Here's how the part is built. I have some questions about the finished solid (model axes, mm). A direction names the side the tool comes from. Round coordinates to 2 decimals unless told otherwise and drop trailing zeros. Order: outer loops, then holes, each group sorted by start corner. A loop starts at its lowest first (then second) coordinate and runs counter-clockwise, first axis right, second up.
```python
from build123d import *

# Parameters (mm, degrees)
CORTAR_EXTRUIR1_REACH   = 95.608
CROQUIS2_R              = 3.5
CROQUIS3_R              = 7
CROQUIS3_R_2            = 3.5
SALIENTE_EXTRUIR1_DEPTH = 6
SALIENTE_EXTRUIR2_START = 3
CROQUIS4_R              = 60.229990605
CROQUIS4_R_2            = 3.5
SALIENTE_EXTRUIR2_DEPTH = 3
CROQUIS5_R              = 5.5
CORTAR_EXTRUIR2_DEPTH   = 6.5
CORTAR_EXTRUIR3_REACH   = 96.128
CORTAR_EXTRUIR4_DEPTH   = 3
CHAFL_N1_SIZE           = 1.5
REDONDEO1_R             = 3


with BuildPart() as part:
    # Croquis1 → Revolución1 (revolve)
    with BuildSketch(Plane.XY, mode=Mode.PRIVATE) as revoluci_n1_sk:
        Polygon((-65.360292755, 76.904610688), (-65.360292755, 76.220570402), (-63.480907514, 76.220570402), (-58.829575529, 89), (0, 89), (0, 91), (-60.229990605, 91), align=None)
    revolve(revoluci_n1_sk.sketch.rotate(Axis((0, 89, 0), (0, 1, 0)), 270), axis=Axis((0, 89, 0), (0, 1, 0)))

    # Croquis2 → Cortar-Extruir1 (cut, up to next)
    with BuildSketch(Plane(origin=(0, 91, 0), x_dir=(1, 0, 0), z_dir=(0, 1, 0)), mode=Mode.PRIVATE) as cortar_extruir1_sk1:
        with Locations(Location((32, 0, 0), (0, 0, 270))):
            Circle(CROQUIS2_R)
    cortar_extruir1_tool1 = extrude(cortar_extruir1_sk1.sketch, amount=-CORTAR_EXTRUIR1_REACH, mode=Mode.PRIVATE) & part.part
    # Croquis2 → Cortar-Extruir1 (cut, up to next)
    with BuildSketch(Plane(origin=(0, 91, 0), x_dir=(1, 0, 0), z_dir=(0, 1, 0)), mode=Mode.PRIVATE) as cortar_extruir1_sk2:
        with Locations(Location((-32, 0, 0), (0, 0, 270))):
            Circle(CROQUIS2_R)
    cortar_extruir1_tool2 = extrude(cortar_extruir1_sk2.sketch, amount=-CORTAR_EXTRUIR1_REACH, mode=Mode.PRIVATE) & part.part
    add(cortar_extruir1_tool1.solids().sort_by_distance((32, 91, 0))[0], mode=Mode.SUBTRACT)
    add(cortar_extruir1_tool2.solids().sort_by_distance((-32, 91, 0))[0], mode=Mode.SUBTRACT)

    # Croquis3 → Saliente-Extruir1 (add)
    # profile 1 of 2: a face of its own
    with BuildSketch(Plane.XZ.offset(-89)):
        with Locations(Location((-32, 0, 0), (0, 0, 90))):
            Circle(CROQUIS3_R)
        with Locations(Location((-32, 0, 0), (0, 0, 90))):
            Circle(CROQUIS3_R_2, mode=Mode.SUBTRACT)
    # profile 2 of 2: a face of its own
    with BuildSketch(Plane.XZ.offset(-89)):
        with Locations(Location((32, 0, 0), (0, 0, 90))):
            Circle(CROQUIS3_R)
        with Locations(Location((32, 0, 0), (0, 0, 90))):
            Circle(CROQUIS3_R_2, mode=Mode.SUBTRACT)
    extrude(amount=SALIENTE_EXTRUIR1_DEPTH)

    # Croquis4 → Saliente-Extruir2 (add)
    with BuildSketch(Plane(origin=(0, 91, 0), x_dir=(1, 0, 0), z_dir=(0, 1, 0)).offset(SALIENTE_EXTRUIR2_START)):
        with Locations(Location((0, 0, 0), (0, 0, 270))):
            Circle(CROQUIS4_R)
        with Locations(Location((32, 0, 0), (0, 0, 270))):
            Circle(CROQUIS4_R_2, mode=Mode.SUBTRACT)
        with Locations(Location((-32, 0, 0), (0, 0, 270))):
            Circle(CROQUIS4_R_2, mode=Mode.SUBTRACT)
    extrude(amount=-SALIENTE_EXTRUIR2_DEPTH)

    # Croquis5 → Cortar-Extruir2 (cut)
    with BuildSketch(Plane(origin=(0, 94, 0), x_dir=(1, 0, 0), z_dir=(0, 1, 0))):
        with Locations(Location((-32, 0, 0), (0, 0, 270))):
            Circle(CROQUIS5_R)
        with Locations(Location((32, 0, 0), (0, 0, 270))):
            Circle(CROQUIS5_R)
    extrude(amount=-CORTAR_EXTRUIR2_DEPTH, mode=Mode.SUBTRACT)

    # Croquis6 → Cortar-Extruir3 (cut, up to next)
    with BuildSketch(Plane(origin=(0, 94, 0), x_dir=(1, 0, 0), z_dir=(0, 1, 0)), mode=Mode.PRIVATE) as cortar_extruir3_sk1:
        with BuildLine():
            Line((-15, -25), (15, -25))
            ThreePointArc((15, -25), (18.535533906, -23.535533906), (20, -20))
            Line((20, -20), (20, 20))
            ThreePointArc((20, 20), (18.535533906, 23.535533906), (15, 25))
            Line((15, 25), (-15, 25))
            ThreePointArc((-15, 25), (-18.535533906, 23.535533906), (-20, 20))
            Line((-20, 20), (-20, -20))
            ThreePointArc((-20, -20), (-18.535533906, -23.535533906), (-15, -25))
        make_face()
    cortar_extruir3_tool1 = extrude(cortar_extruir3_sk1.sketch, amount=-CORTAR_EXTRUIR3_REACH, mode=Mode.PRIVATE) & part.part
    add(cortar_extruir3_tool1.solids().sort_by_distance((0, 94, 0))[0], mode=Mode.SUBTRACT)

    # Croquis7 → Cortar-Extruir4 (cut)
    with BuildSketch(Plane(origin=(0, 94, 0), x_dir=(1, 0, 0), z_dir=(0, 1, 0))):
        with BuildLine():
            Line((-15, -27), (15, -27))
            ThreePointArc((15, -27), (19.949747468, -24.949747468), (22, -20))
            Line((22, -20), (22, 20))
            ThreePointArc((22, 20), (19.949747468, 24.949747468), (15, 27))
            Line((15, 27), (-15, 27))
            ThreePointArc((-15, 27), (-19.949747468, 24.949747468), (-22, 20))
            Line((-22, 20), (-22, -20))
            ThreePointArc((-22, -20), (-19.949747468, -24.949747468), (-15, -27))
        make_face()
    extrude(amount=-CORTAR_EXTRUIR4_DEPTH, mode=Mode.SUBTRACT)

    # Chaflán1
    chafl_n1_edges = [part.edges().sort_by_distance(p)[0] for p in [
        (0, 91, 25),
        (-18.535533906, 91, 23.535533906),
        (-20, 91, 0),
        (-18.535533906, 91, -23.535533906),
        (0, 91, -25),
        (18.535533906, 91, -23.535533906),
        (20, 91, 0),
        (18.535533906, 91, 23.535533906),
    ]]
    chamfer(chafl_n1_edges, length=CHAFL_N1_SIZE)

    # Redondeo1
    redondeo1_edges = [part.edges().sort_by_distance(p)[0] for p in [
        (0, 94, -60.229990605),
    ]]
    fillet(redondeo1_edges, radius=REDONDEO1_R - 0.0001)  # a hair under: the kernel refuses the full size


solid = part.part
```
1. If we section it at B-B, the plane y = 84.75: Write out the boundary of the cut face in (x, z).
Evaluation:
outline: circle Ø125.01 at (0, 0); circle Ø14 at (-32, 0); circle Ø14 at (32, 0); hole circle Ø120.75 at (0, 0); hole circle Ø7 at (-32, 0); hole circle Ø7 at (32, 0)
2. If we mould it in two halves opening along Z, with no side actions, what happens to faces 4 (the conical face through (-60.036, 90.118, 7.883)), 5 (the flat face through (-34, 76.221, 54)), 6 (the cylindrical face through (20, 92.5, -24.9))? For each: released by +Z, released by -Z, zero draft, split by the parting line, or undercut.
Evaluation:
face 4: split by the parting line
face 5: zero draft
face 6: undercut
3. I'm going to push flat-ended pins straight in: P1, Ø1.5, axis at x = -5.5, y = 92.5, coming from the +Z side; P2, Ø4, axis at y = 79, z = 24.5, coming from the -X side; P3, Ø5, axis at y = 85.5, z = -23, coming from the +X side; P4, Ø4, axis at x = 32, z = 0, coming from the -Y side. Where does each tip first touch, or does it pass through?
Evaluation:
P1: stops at z = 59.89
P2: stops at x = -60.88
P3: stops at x = 59.18
P4: passes through
4. If we section it at C-C, the plane z = 0: State how many separate pieces and enclosed holes the cut face has, and give its area (3 significant figures).
Evaluation:
separate pieces: 4
enclosed holes: 0
area: 402 mm2
5. On a 3-axis mill with a long thin cutter (end or side, diameter ignored), from which of +Z, -Z, +X, -X, +Y, -Y can I reach the whole of each face in a straight line? I mean faces 1 (the flat face through (-0.8, 89, -25.3)), 2 (the conical face through (-18.78, 89.906, 23.865)), 3 (the cylindrical face through (18.5, 89.25, 23.57)). Say none if no direction works.
Evaluation:
face 1: -Y
face 2: +Y
face 3: +Y, -Y
6. I need wall thicknesses on probe 1 along Z at (x, y) = (32, 86); probe 2 along Z at (x, y) = (32, 86.1); probe 3 along X at (y, z) = (92.5, 0). Which ranges of each line are inside material? Lowest first, please.
Evaluation:
probe 1: z = -53.16 to -50.66, -7 to -3.5, 3.5 to 7, 50.66 to 53.16
probe 2: z = -53.12 to -50.62, -7 to -3.5, 3.5 to 7, 50.62 to 53.12
probe 3: x = -59.83 to -37.5, -26.5 to -22, 22 to 26.5, 37.5 to 59.83
